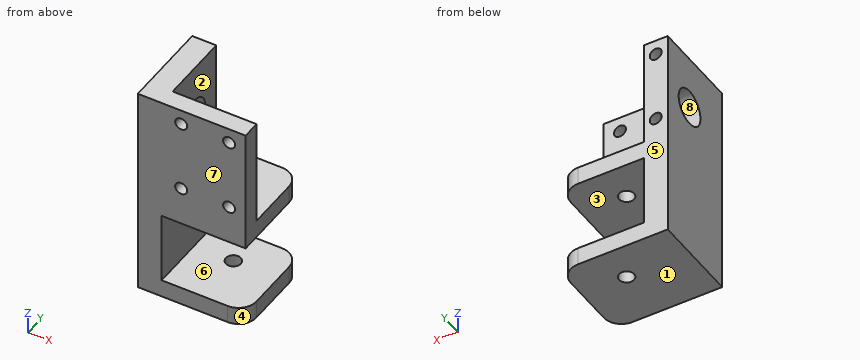
from build123d import *

# Parameters (mm, degrees)
EXTRUDE_2_DEPTH     = 15
FILLET_1_R          = 3
CUT_EXTRUDE_1_REACH = 31.547
SKETCH_4_R          = 1.25
EXTRUDE_START       = -12
SKETCH_5_W          = 18
SKETCH_5_H          = 18
EXTRUDE_3_DEPTH     = 3
SKETCH_6_W          = 4
SKETCH_6_H          = 18
EXTRUDE_5_DEPTH     = 12
SKETCH_8_R          = 3
CUT_EXTRUDE_2_DEPTH = 28.294688128
SKETCH_9_R          = 1
CUT_EXTRUDE_3_DEPTH = 29.142494559
SKETCH_10_R         = 1
CUT_EXTRUDE_4_DEPTH = 5


with BuildPart() as part:
    # 草图2 → 凸台-拉伸2 (new body)
    with BuildSketch(Plane(origin=(0, 0, 0), x_dir=(1, 0, 0), z_dir=(0, 1, 0))):
        Polygon((18, 0), (0, 0), (0, 18), (18, 18), (18, 15), (4, 15), (4, 3), (18, 3), align=None)
    extrude(amount=EXTRUDE_2_DEPTH)

    # 圆角1
    fillet_1_edges = [part.edges().sort_by_distance(p)[0] for p in [
        (18, 0, -16.5),
        (18, 15, -16.5),
        (18, 15, -1.5),
    ]]
    fillet(fillet_1_edges, radius=FILLET_1_R)

    # 切除-拉伸1: up to this face of the body (flat: up to its plane)
    cut_extrude_1_end = Plane(part.part.faces().sort_by_distance((8.939983645, 7.450791047, 0))[0])
    # 草图4 → 切除-拉伸1 (cut, up to the picked face)
    with BuildSketch(Plane(origin=(0, 0, -18), x_dir=(-1, 0, 0), z_dir=(0, 0, -1)), mode=Mode.PRIVATE) as cut_extrude_1_sk1:
        with Locations((-10.5, 9)):
            Circle(SKETCH_4_R)
    cut_extrude_1_tool1 = split(extrude(cut_extrude_1_sk1.sketch, amount=-CUT_EXTRUDE_1_REACH, mode=Mode.PRIVATE), bisect_by=cut_extrude_1_end, keep=Keep.BOTH, mode=Mode.PRIVATE)
    add(cut_extrude_1_tool1.solids().sort_by(Axis((10.5, 9, -18), (0, 0, 1)))[0], mode=Mode.SUBTRACT)

    # 草图5 → 凸台-拉伸3 (add)
    with BuildSketch(Plane(origin=(0, 15, 0), x_dir=(1, 0, 0), z_dir=(0, 1, 0)).offset(EXTRUDE_START)):
        with Locations((9, -9)):
            Rectangle(SKETCH_5_W, SKETCH_5_H)
    extrude(amount=-EXTRUDE_3_DEPTH)

    # 草图6 → 凸台-拉伸5 (add)
    with BuildSketch(Plane(origin=(0, 3, 0), x_dir=(1, 0, 0), z_dir=(0, 1, 0))):
        with Locations((2, -9)):
            Rectangle(SKETCH_6_W, SKETCH_6_H)
    extrude(amount=EXTRUDE_5_DEPTH)

    # 草图8 → 切除-拉伸2 (cut, through all)
    with BuildSketch(Plane(origin=(4, 0, 0), x_dir=(0, 0, -1), z_dir=(1, 0, 0))):
        with Locations((-9, 9)):
            Circle(SKETCH_8_R)
    extrude(amount=-CUT_EXTRUDE_2_DEPTH, mode=Mode.SUBTRACT)

    # 草图9 → 切除-拉伸3 (cut, through all)
    with BuildSketch(Plane(origin=(0, 3, 0), x_dir=(1, 0, 0), z_dir=(0, 1, 0))):
        with Locations(Location((7.25, -15.5, 0), (0, 0, 270))):
            Circle(SKETCH_9_R)
        with Locations(Location((15.25, -15.5, 0), (0, 0, 270))):
            Circle(SKETCH_9_R)
        with Locations(Location((7.25, -3.5, 0), (0, 0, 270))):
            Circle(SKETCH_9_R)
        with Locations(Location((15.25, -3.5, 0), (0, 0, 270))):
            Circle(SKETCH_9_R)
    extrude(amount=-CUT_EXTRUDE_3_DEPTH, mode=Mode.SUBTRACT)

    # 草图10 → 切除-拉伸4 (cut)
    with BuildSketch(Plane(origin=(0, 15, 0), x_dir=(1, 0, 0), z_dir=(0, 1, 0))):
        with Locations(Location((2, -15.5, 0), (0, 0, 270))):
            Circle(SKETCH_10_R)
        with Locations(Location((2, -3.5, 0), (0, 0, 270))):
            Circle(SKETCH_10_R)
    extrude(amount=-CUT_EXTRUDE_4_DEPTH, mode=Mode.SUBTRACT)


solid = part.part
Verification items for the finished model (mm, model axes). Face numbers are marked on the shaded views. A direction names the side the tool comes from. Round coordinates to 2 decimals unless told otherwise and drop trailing zeros. Loops run counter-clockwise (first coordinate to the right, second up) from the corner with the lowest first, then second, coordinate; pieces in that order, holes last. Notation, with made-up numbers: (58, 24.5) - (107, 24.5) arc R25 cw to (107, 49.5) - close; hole circle Ø11 at (49, 41.5). An arc over 180 degrees is marked (long way). Use a Markdown table: item, result. Add a question column.
1. Access from +Z, -Z, +X, -X, +Y, -Y to the whole of each face (thin tool, end or side, straight path). Record for the marked faces 1, 2, 3 and 4.
2. Gauge pin test, flat ends, axial feed: pin 1 (0.6 mm diameter, centred on x = 2, z = 15.5, fed in from +Y); pin 2 (8 mm diameter, centred on y = 5, z = -7.5, fed in from +X); pin 3 (3 mm diameter, centred on x = 8, y = 5, fed in from +Z). Record the tip position at first contact, or that the pin passes through.
3. Release check for a two-part mould opening along Y. For the marked faces 5, 6, 7 and 8 record: released by +Y, released by -Y, zero draft, split by the parting line, or undercut.
4. Thickness scan on probe 1 along X at (y, z) = (2.15, 15.5); probe 2 along X at (y, z) = (12.65, 15.5); probe 3 along Z at (x, y) = (7.75, 2.5). Record the ranges inside material, lowest first. Write a range as [from, to].
5. Section check D-D, the plane x = 7.25. Record the boundary of the cut face in (y, z), plus the area to 3 significant figures.
6. Section check C-C, the plane x = 3.5. Record the boundary of the cut face in (y, z), plus the area to 3 significant figures.
7. Section check A-A, the plane y = 9. Record the boundary of the cut face in (x, z).
8. Section check B-B, the plane z = 15.5. Record the boundary of the cut face in (x, y).
Checks:
| question | item | result |
|---|---|---|
| 1 | face 1 | -Z, +X, -X, +Y, -Y |
| 1 | face 2 | +Z, +X, +Y |
| 1 | face 3 | +X, +Y, -Y |
| 1 | face 4 | -Z, +X, -Y |
| 2 | pin 1 | stops at y = 10 |
| 2 | pin 2 | stops at x = 4 |
| 2 | pin 3 | stops at z = 0 |
| 3 | face 5 | released by +Y |
| 3 | face 6 | zero draft |
| 3 | face 7 | released by -Y |
| 3 | face 8 | undercut |
| 4 | probe 1 | x = [0, 6.25], [8.25, 14.25], [16.25, 18] |
| 4 | probe 2 | x = [0, 1], [3, 4] |
| 4 | probe 3 | z = [-18, -15], [-3, 2.63], [4.37, 14.63], [16.37, 18] |
| 5 | outline | (0, -18) - (15, -18) - (15, -15) - (0, -15) - close; (0, -3) - (15, -3) - (15, 0) - (3, 0) - (3, 2.5) - (0, 2.5) - close; (0, 4.5) - (3, 4.5) - (3, 14.5) - (0, 14.5) - close; (0, 16.5) - (3, 16.5) - (3, 18) - (0, 18) - close |
| 5 | area | 132 mm^2 |
| 6 | outline | (0, -18) - (15, -18) - (15, 18) - (0, 18) - close; hole circle Ø6 at (9, 9) |
| 6 | area | 512 mm^2 |
| 7 | outline | (0, -18) - (9.25, -18) - (9.25, -15) - (4, -15) - (4, -3) - (9.25, -3) - (9.25, 0) - (4, 0) - (4, 6) - (0, 6) - close; (0, 12) - (4, 12) - (4, 18) - (0, 18) - close; (11.75, -18) - (18, -18) - (18, -15) - (11.75, -15) - close; (11.75, -3) - (18, -3) - (18, 0) - (11.75, 0) - close |
| 8 | outline | (0, 0) - (6.25, 0) - (6.25, 3) - (4, 3) - (4, 15) - (3, 15) - (3, 10) - (1, 10) - (1, 15) - (0, 15) - close; (8.25, 0) - (14.25, 0) - (14.25, 3) - (8.25, 3) - close; (16.25, 0) - (18, 0) - (18, 3) - (16.25, 3) - close |
